Can you work these out from the drawing? Everything is in mm from the part's minimum corner. A direction names the side the tool comes from. Give positions to 0.01 mm unless a question says otherwise; leave off trailing zeros. Loops run counter-clockwise (first coordinate to the right, second up) from the corner with the lowest first, then second, coordinate; pieces in that order, holes last. Notation, with made-up numbers: (30, 89.5) -> (74, 89.5) arc R11 ccw to (74, 99.5) -> close; hole circle Ø10 at (-13.5, 4). An arc over 180 degrees is marked (long way). Return JSON: item names as keys, results as strings. Group by question number.
Q1. Suppose I cut it at C-C, the plane x = 5.75. Please give me the cut outline in (y, z) (1 decimal).
Q2. Which directions (+Z, -Z, +X, -X, +Y, -Y) give clear straight access to the entire face, cutting with the end or side of a thin tool? Please do the marked faces 1, 2 and 3.
Q3. I need wall thicknesses on line 1 along X through (y, z) = (15.5, 35) (1 decimal); line 2 along X through (y, z) = (27, 8); line 3 along Y through (x, z) = (6.5, 21). Which ranges of each line are inside material? Lowest first, please. Write a range as [from, to].
Q4. Suppose I cut it at D-D, the plane x = 15.25. Please give me the cut outline in (y, z) (1 decimal), and give its area (3 significant figures).
Q5. Will these pins go through, and if not, where does the flat tip stop? pin 1 (5 mm diameter, centred on x = 20.5, y = 5, fed in from +Z); pin 2 (5 mm diameter, centred on y = 3.937, z = 32.512, fed in from -X); pin 3 (4 mm diameter, centred on x = 4.5, y = 20.5, fed in from +Z).
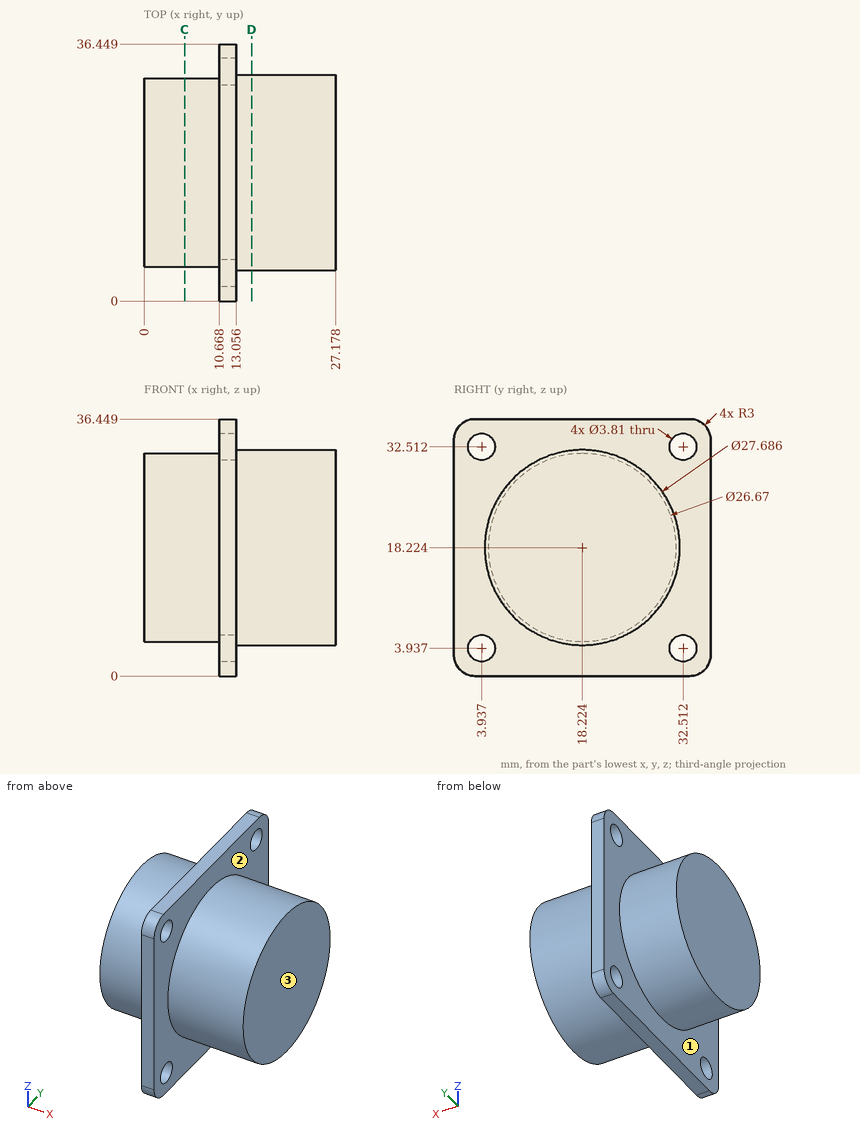
Ans:
{
 "1": {"outline": "circle Ø26.7 at (18.2, 18.2)"},
 "2": {"face 1": "-X", "face 2": "+X", "face 3": "+Z, -Z, +X, +Y, -Y"},
 "3": {"line 1": "x = [10.7, 13.1]", "line 2": "x = [10.67, 27.18]", "line 3": "y = [5.18, 31.27]"},
 "4": {"outline": "circle Ø27.7 at (18.2, 18.2)", "area": "602 mm^2"},
 "5": {"pin 1": "stops at z = 26.98", "pin 2": "stops at x = 10.67", "pin 3": "stops at z = 31.56"}
}
